Check sheet for the modelled part. Datum: model origin and axes. Units: mm. Round coordinates to 2 decimals unless told otherwise and drop trailing zeros. Loops run counter-clockwise (first coordinate to the right, second up) from the corner with the lowest first, then second, coordinate; pieces in that order, holes last. Notation, with made-up numbers: (42, -15) - (90, -15) arc R30 cw to (90, 22) - close; hole circle Ø3 at (-9, -22.75). An arc over 180 degrees is marked (long way). Answer in a Markdown table with one row per item. Add a question column.
(1) Thickness scan on line 1 along X through (y, z) = (1.7, -0.35); line 2 along X through (y, z) = (-0.85, -0.2); line 3 along Y through (x, z) = (2, 0). Record the ranges inside material, lowest first.
(2) Gauge pin test, flat ends, axial feed: pin 1 (1 mm diameter, centred on x = 1.5, y = 1.5, fed in from -Z); pin 2 (2 mm diameter, centred on x = 2.5, y = 1, fed in from +Z); pin 3 (1.2 mm diameter, centred on y = -0.5, z = -1, fed in from +X). Record the tip position at first contact, or that the pin passes through.
(3) Cross-section at A-A on x = 1.75. Enter the section's corners in (y, z).
from build123d import *

# Parameters (mm, degrees)
FILLET1_R                = 0.1
RECPAT_COUNT             = 2
RECPAT_ANGLE             = 90
THDSCHPAT_COUNT          = 19
THDSCHPAT_PITCH          = 0.4
ESBO_O1_R                = 2.4
RESSALTO_EXTRUS_O1_DEPTH = 0.5
SCALE1_SCALE             = 0.8


with BuildPart() as part:
    # BodySke → Base-Revolve (revolve)
    with BuildSketch(Plane.XY, mode=Mode.PRIVATE) as base_revolve_sk:
        with BuildLine():
            Line((1.6, 1), (1.6, 2))
            Line((1.6, 2), (1.1, 2))
            ThreePointArc((1.1, 2), (0.688403396, 1.885994341), (0.394117647, 1.576470588))
            ThreePointArc((0.394117647, 1.576470588), (0.100022625, 0.812494344), (0, 0))
            Line((0, 0), (9.6, 0))
            Line((9.6, 0), (9.6, 1))
            Line((9.6, 1), (1.6, 1))
        make_face()
    revolve(base_revolve_sk.sketch.rotate(Axis((1.1, 0, 0), (1, 0, 0)), 90), axis=Axis((1.1, 0, 0), (1, 0, 0)))

    # Fillet1
    fillet1_edges = [part.edges().sort_by_distance(p)[0] for p in [
        (1.6, 0, -1),
    ]]
    fillet(fillet1_edges, radius=FILLET1_R)

    # Sketch3 → Recess section 0
    with BuildSketch(Plane(origin=(0, 0, 0), x_dir=(0, 0, -1), z_dir=(1, 0, 0))):
        with BuildLine():
            Line((0.24, -1.05), (-0.24, -1.05))
            Line((-0.24, -1.05), (-0.24, 1.05))
            Line((-0.24, 1.05), (0.24, 1.05))
            Line((0.24, 1.05), (0.24, -1.05))
        make_face()
    # Sketch4 → Recess section 1
    with BuildSketch(Plane(origin=(1.42, 0, 0), x_dir=(0, 0, -1), z_dir=(1, 0, 0))):
        with BuildLine():
            Line((0.24, -0.342014235), (-0.24, -0.342014235))
            Line((-0.24, -0.342014235), (-0.24, 0.342014235))
            Line((-0.24, 0.342014235), (0.24, 0.342014235))
            Line((0.24, 0.342014235), (0.24, -0.342014235))
        make_face()
    recess = loft(mode=Mode.SUBTRACT)

    # RecPat: Recess ×2 about axis
    recpat_axis = Axis((0, 0, 0), (1, 0, 0))
    for i in range(1, RECPAT_COUNT):
        add(recess.rotate(recpat_axis, i * RECPAT_ANGLE / (RECPAT_COUNT - 1)), mode=Mode.SUBTRACT)

    # RecCorSke → RecessCore (revolve, cut)
    with BuildSketch(Plane.XY, mode=Mode.PRIVATE) as recesscore_sk:
        Polygon((0, 0), (0, 0.454796073), (1.42, 0.3555), (1.535508952, 0), align=None)
    revolve(recesscore_sk.sketch.rotate(Axis((-3.175, 0, 0), (1, 0, 0)), 13.849905977), axis=Axis((-3.175, 0, 0), (1, 0, 0)), mode=Mode.SUBTRACT)

    # ThdSchSke → ThreadSchematic (revolve, cut)
    with BuildSketch(Plane.XY, mode=Mode.PRIVATE) as threadschematic_sk:
        Polygon((2.4, -0.774), (2.241753096, -1), (2.241753096, -1.25), (2.558246904, -1.25), (2.558246904, -1), align=None)
    threadschematic = revolve(threadschematic_sk.sketch.rotate(Axis((-3.175, 0, 0), (1, 0, 0)), 270), axis=Axis((-3.175, 0, 0), (1, 0, 0)), mode=Mode.SUBTRACT)

    # ThdSchPat: ThreadSchematic ×19
    with Locations(*[(i * THDSCHPAT_PITCH, 0, 0) for i in range(1, THDSCHPAT_COUNT)]):
        add(threadschematic, mode=Mode.SUBTRACT)

    # Esboço1 → Ressalto-extrusão1 (add)
    with BuildSketch(Plane(origin=(1.6, 0, 0), x_dir=(0, 0, -1), z_dir=(1, 0, 0))):
        Circle(ESBO_O1_R)
    extrude(amount=-RESSALTO_EXTRUS_O1_DEPTH)

    # Esboço2 → Corte-Revolução1 (revolve, cut)
    with BuildSketch(Plane(origin=(0, 0, 0), x_dir=(1, 0, 0), z_dir=(0, 1, 0)), mode=Mode.PRIVATE) as corte_revolu_o1_sk:
        Polygon((9.6, 0.3), (8.1, 1), (9.6, 1), align=None)
    revolve(corte_revolu_o1_sk.sketch.rotate(Axis((0, 0, 0), (1, 0, 0)), 270), axis=Axis((0, 0, 0), (1, 0, 0)), mode=Mode.SUBTRACT)


with BuildPart() as part_1:
    # Scale1: scaled about (3.259576081, 1.9e-08, -1.5e-08)
    add(part.part.scale(SCALE1_SCALE).moved(Location((0.651915216, 4e-09, -3e-09))))


solid = part_1.part
Answers:
| question | item | result |
|---|---|---|
| 1 | line 1 | x = 1.53 to 1.93 |
| 1 | line 2 | x = 0.8 to 1.93 |
| 1 | line 3 | y = -0.8 to 0.8 |
| 2 | pin 1 | stops at z = -1.64 |
| 2 | pin 2 | stops at z = 1.91 |
| 2 | pin 3 | stops at x = 7.74 |
| 3 | outline | circle Ø3.84 at (0, 0) |
